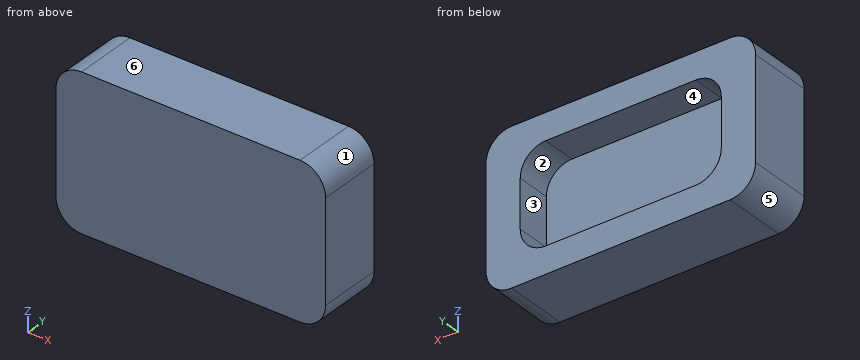
```python
from build123d import *

# Parameters (mm, degrees)
F1_DEPTH = 25
F3_DEPTH = 13.5


with BuildPart() as f1:
    # F0 (on Front) → F1 (new body)
    with BuildSketch(Plane.XZ):
        with BuildLine():
            ThreePointArc((-52.798297, -19.829547), (-49.869365, -26.900615), (-42.798297, -29.829547))
            Line((-42.798297, -29.829547), (42.798297, -29.829547))
            ThreePointArc((42.798297, -29.829547), (49.869365, -26.900615), (52.798297, -19.829547))
            Line((52.798297, -19.829547), (52.798297, 19.829547))
            ThreePointArc((52.798297, 19.829547), (49.869365, 26.900615), (42.798297, 29.829547))
            Line((42.798297, 29.829547), (-42.798297, 29.829547))
            ThreePointArc((-42.798297, 29.829547), (-49.869365, 26.900615), (-52.798297, 19.829547))
            Line((-52.798297, 19.829547), (-52.798297, -19.829547))
        make_face()
    extrude(amount=F1_DEPTH)

    # F2 (on face) → F3 (cut)
    with BuildSketch(Plane(origin=(0, 0, 0), x_dir=(-1, 0, 0), z_dir=(0, 1, 0))):
        with BuildLine():
            ThreePointArc((-39.375003, -9.389205), (-36.446071, -16.460272), (-29.375003, -19.389205))
            Line((-29.375003, -19.389205), (29.375003, -19.389205))
            ThreePointArc((29.375003, -19.389205), (36.446071, -16.460272), (39.375003, -9.389205))
            Line((39.375003, -9.389205), (39.375003, 9.389205))
            ThreePointArc((39.375003, 9.389205), (36.446071, 16.460272), (29.375003, 19.389205))
            Line((29.375003, 19.389205), (-29.375003, 19.389205))
            ThreePointArc((-29.375003, 19.389205), (-36.446071, 16.460272), (-39.375003, 9.389205))
            Line((-39.375003, 9.389205), (-39.375003, -9.389205))
        make_face()
    extrude(amount=-F3_DEPTH, mode=Mode.SUBTRACT)


solid = f1.part
```
Geometry: final body of the model. Coordinates: model frame, mm. Face numbers are marked on the shaded views. A direction names the side the tool comes from. Round coordinates to 2 decimals unless told otherwise and drop trailing zeros. Order: outer loops, then holes, each group sorted by start corner. A loop starts at its lowest first (then second) coordinate and runs counter-clockwise, first axis right, second up. Notation, with made-up numbers: (32.5, 54.5) -> (59.5, 54.5) arc R34 cw to (59.5, 86.5) -> close; hole circle Ø2 at (5, 33). An arc over 180 degrees is marked (long way). Write each question's results on one line, items separated by ' | '.
Q1. Access query for the marked faces 1 and 2. Directions: +Z, -Z, +X, -X, +Y, -Y. A direction counts if a zero-diameter tool reaches every point of the face in a straight line with its end or side. Return the directions, or none.
Response values:
face 1: +Z, +X, +Y, -Y | face 2: +Y
Q2. Ray query, line 1 along X through (y, z) = (-3, -5.5) (3 decimals); line 2 along Z through (x, y) = (-23, -4); line 3 along Y through (x, z) = (-30, 18.5). Return the intervals inside material, ascending.
Response values:
line 1: -52.798 to -39.375, 39.375 to 52.798 | line 2: -29.83 to -19.39, 19.39 to 29.83 | line 3: -25 to -13.5
Q3. Section query C-C (z = 7). Output: boundary loops of the cut face in (x, y) (3 decimals).
Response values:
outline: (-52.798, -25) -> (52.798, -25) -> (52.798, 0) -> (39.375, 0) -> (39.375, -13.5) -> (-39.375, -13.5) -> (-39.375, 0) -> (-52.798, 0) -> close
Q4. Section query D-D (z = -25.5). Output: boundary loops of the cut face in (x, y).
Response values:
outline: (-51.04, -25) -> (51.04, -25) -> (51.04, 0) -> (-51.04, 0) -> close
Q5. Section query B-B (x = 20). Output: boundary loops of the cut face in (y, z), and give its area (3 significant figures).
Response values:
outline: (-25, -29.83) -> (0, -29.83) -> (0, -19.39) -> (-13.5, -19.39) -> (-13.5, 19.39) -> (0, 19.39) -> (0, 29.83) -> (-25, 29.83) -> close | area: 968 mm²
Q6. Pin query (flat end, axial travel): pin 1 Ø4 at (y, z) = (-11.5, 22) entering from +X. Return the tip coordinate at first contact, or that it passes through.
Response values:
pin 1: x = 52.8
Q7. Section query A-A (y = -12). Output: boundary loops of the cut face in (x, z) (3 decimals), and give its area (3 significant figures).
Response values:
outline: (-52.798, -19.83) arc R10 ccw to (-42.798, -29.83) -> (42.798, -29.83) arc R10 ccw to (52.798, -19.83) -> (52.798, 19.83) arc R10 ccw to (42.798, 29.83) -> (-42.798, 29.83) arc R10 ccw to (-52.798, 19.83) -> close; hole (-39.375, -9.389) arc R10 ccw to (-29.375, -19.389) -> (29.375, -19.389) arc R10 ccw to (39.375, -9.389) -> (39.375, 9.389) arc R10 ccw to (29.375, 19.389) -> (-29.375, 19.389) arc R10 ccw to (-39.375, 9.389) -> close | area: 3,250 mm²
Q8. Pull-direction query (X, two-part tool) for the marked faces 3, 4, 5 and 6; classes: released by +X, released by -X, zero draft, split by the parting line, or undercut.
Response values:
face 3: undercut | face 4: undercut | face 5: released by -X | face 6: zero draft
